Autodesk Inventor part; units mm, degrees
ref_plane "YZ Plane" through (0, 0, 0) normal (1, 0, 0) x (0, 1, 0)
ref_plane "XZ Plane" through (0, 0, 0) normal (0, 1, 0) x (-1, 0, 0)
ref_plane "XY Plane" through (0, 0, 0) normal (0, 0, 1) x (1, 0, 0)
sketch "Sketch1" plane through (0, 0, 0) normal (0, 0, 1) x (1, 0, 0)
  line L0 (0, 0) -> (0, 7)
  line L1 (0, 7) -> (6, 7)
  line L2 (6, 7) -> (6, 5)
  line L3 (6, 5) -> (11, 5)
  line L4 (11, 5) -> (11, 0)
  line L5 (11, 0) -> (0, 0)
  dimension "d0" = 5
  dimension "d1" = 6
  dimension "d2" = 10
  dimension "d3" = 14
revolve "Revolution1" add sketch "Sketch1" angle 360 about axis through (11, 0, 0) along (-1, 0, 0)
sketch "Sketch2" plane through (0, 0, 0) normal (-1, 0, 0) x (0, 0, 1)
  circle A0 centre (0, 0) radius 7
  point P0 (0, 0)
hole "Hole1" at (0, 0, 0) direction (1, 0, 0) diameter 4.134 depth 9
properties part number "1 part 16"
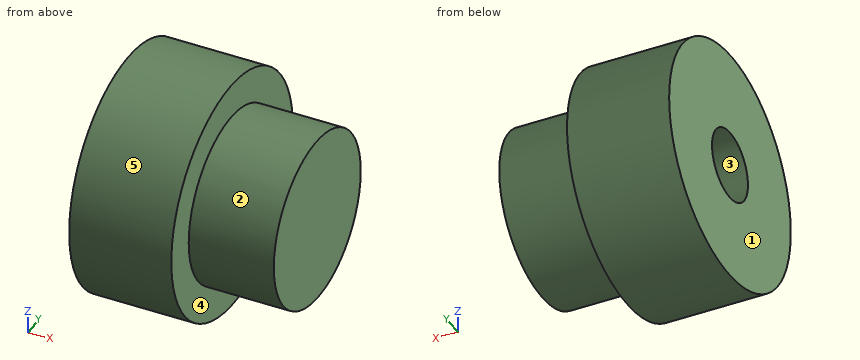
Check sheet for the modelled part. Datum: model origin and axes. Units: mm. Face numbers are marked on the shaded views. A direction names the side the tool comes from. Coordinates: 2 decimals unless noted, no trailing zeros. Write each loop counter-clockwise with the first axis right and the second up, starting at its lowest first coordinate (ties: lowest second). Pieces come first, ordered by that corner, then holes. Notation, with made-up numbers: (-33, 19.5) -> (25, 19.5) arc R14 ccw to (25, 43.5) -> close; hole circle Ø11 at (59.25, 28). An arc over 180 degrees is marked (long way). Use a Markdown table: item, result.
1. Tool access check on the marked faces 1 and 2. Record the directions out of +Z, -Z, +X, -X, +Y, -Y that give a thin tool (end or side, any length) a straight path to the whole face; none if there is none.
Reported:
| item | result |
|---|---|
| face 1 | +Z, -Z, -X, +Y, -Y |
| face 2 | +X |
2. Scan lines: line 1 along Y through (x, z) = (3.5, 0); line 2 along Y through (x, z) = (6.25, 0). Record each from-to range of solid material in increasing order.
Reported:
| item | result |
|---|---|
| line 1 | y = -7 to -2.07, 2.07 to 7 |
| line 2 | y = -5 to -2.07, 2.07 to 5 |
3. Sectioned sample at C-C (x = 6.5). Enter the section's corners in (y, z).
Reported:
| item | result |
|---|---|
| outline | circle Ø10 at (0, 0); hole circle Ø4.13 at (0, 0) |
4. Sectioned sample at A-A (z = 0). Enter the section's corners in (x, y), plus the area to 3 significant figures.
Reported:
| item | result |
|---|---|
| outline | (0, -7) -> (6, -7) -> (6, -5) -> (11, -5) -> (11, 5) -> (6, 5) -> (6, 7) -> (0, 7) -> (0, 2.07) -> (9, 2.07) -> (9, -2.07) -> (0, -2.07) -> close |
| area | 96.8 mm2 |
5. Release check for a two-part mould opening along Z. For the marked faces 3, 4 and 5 record: pulls with the +Z half, pulls with the -Z half, needs draft (parallel to the pull), parting line crosses it, or undercut.
Reported:
| item | result |
|---|---|
| face 3 | undercut |
| face 4 | needs draft |
| face 5 | parting line crosses it |
6. Go/stop test with flat-tipped pins: pin 1 Ø6 at (x, z) = (3, 3) entering from +Y; pin 2 Ø3.5 at (y, z) = (0, 0) entering from -X; pin 3 Ø5 at (x, y) = (3.5, -3.5) entering from +Z; pin 4 Ø2 at (x, z) = (8, -1) entering from -Y. Record where each tip stops, or that it passes through.
Reported:
| item | result |
|---|---|
| pin 1 | stops at y = 7 |
| pin 2 | stops at x = 9 |
| pin 3 | stops at z = 6.93 |
| pin 4 | stops at y = -5 |
7. Sectioned sample at D-D (x = 10.25). Enter the section's corners in (y, z), plus the area to 3 significant figures.
Reported:
| item | result |
|---|---|
| outline | circle Ø10 at (0, 0) |
| area | 78.5 mm2 |
